from build123d import *

# Parameters (mm, degrees)
SKETCH1_W           = 190.5
SKETCH1_H           = 190.5
BOSS_EXTRUDE1_DEPTH = 9.525
SKETCH2_W           = 38.1
SKETCH2_H           = 9.525
CUT_EXTRUDE1_DEPTH  = 9.525
SKETCH3_W           = 38.1
SKETCH3_H           = 9.525
CUT_EXTRUDE2_DEPTH  = 9.525
SKETCH4_W           = 9.525
SKETCH4_H           = 28.575
CUT_EXTRUDE3_DEPTH  = 9.525
SKETCH5_W           = 9.525
SKETCH5_H           = 38.1
CUT_EXTRUDE4_DEPTH  = 9.525
SKETCH6_W           = 9.525
SKETCH6_H           = 28.575
CUT_EXTRUDE5_DEPTH  = 9.525
SKETCH7_W           = 38.1
SKETCH7_H           = 9.525
CUT_EXTRUDE6_DEPTH  = 9.525
SKETCH8_W           = 38.1
SKETCH8_H           = 9.525
CUT_EXTRUDE7_DEPTH  = 9.525
SKETCH9_W           = 9.525
SKETCH9_H           = 28.575
CUT_EXTRUDE8_DEPTH  = 38.1
SKETCH10_W          = 9.525
SKETCH10_H          = 38.1
CUT_EXTRUDE9_DEPTH  = 9.525
SKETCH11_W          = 9.525
SKETCH11_H          = 28.575
CUT_EXTRUDE10_DEPTH = 9.525
SKETCH12_W          = 25.4
SKETCH12_H          = 3.175
CUT_EXTRUDE11_DEPTH = 12.7
SKETCH15_W          = 6.35
SKETCH15_H          = 9.525
CUT_EXTRUDE14_DEPTH = 214.194785552
SKETCH19_W          = 6.35
SKETCH19_H          = 38.1
SKETCH19_H_2        = 9.525
CUT_EXTRUDE16_DEPTH = 214.194785552
SKETCH16_W          = 6.35
SKETCH16_H          = 38.1
SKETCH16_H_2        = 9.525
CUT_EXTRUDE15_DEPTH = 209.566482942


with BuildPart() as part:
    # Sketch1 → Boss-Extrude1 (new body)
    with BuildSketch(Plane(origin=(0, 0, 0), x_dir=(1, 0, 0), z_dir=(0, 1, 0))):
        with Locations((61.628840928, 48.799714441)):
            Rectangle(SKETCH1_W, SKETCH1_H)
    extrude(amount=BOSS_EXTRUDE1_DEPTH)

    # Sketch2 → Cut-Extrude1 (cut)
    with BuildSketch(Plane(origin=(0, 9.525, 0), x_dir=(1, 0, 0), z_dir=(0, 1, 0))):
        with Locations((99.728840928, -41.687785559)):
            Rectangle(SKETCH2_W, SKETCH2_H)
    extrude(amount=-CUT_EXTRUDE1_DEPTH, mode=Mode.SUBTRACT)

    # Sketch3 → Cut-Extrude2 (cut)
    with BuildSketch(Plane(origin=(0, 9.525, 0), x_dir=(1, 0, 0), z_dir=(0, 1, 0))):
        with Locations((23.528840928, -41.687785559)):
            Rectangle(SKETCH3_W, SKETCH3_H)
    extrude(amount=-CUT_EXTRUDE2_DEPTH, mode=Mode.SUBTRACT)

    # Sketch4 → Cut-Extrude3 (cut)
    with BuildSketch(Plane(origin=(0, 9.525, 0), x_dir=(1, 0, 0), z_dir=(0, 1, 0))):
        with Locations((152.116340928, -22.637785559)):
            Rectangle(SKETCH4_W, SKETCH4_H)
    extrude(amount=-CUT_EXTRUDE3_DEPTH, mode=Mode.SUBTRACT)

    # Sketch5 → Cut-Extrude4 (cut)
    with BuildSketch(Plane(origin=(0, 9.525, 0), x_dir=(1, 0, 0), z_dir=(0, 1, 0))):
        with Locations((152.116340928, 48.799714441)):
            Rectangle(SKETCH5_W, SKETCH5_H)
    extrude(amount=-CUT_EXTRUDE4_DEPTH, mode=Mode.SUBTRACT)

    # Sketch6 → Cut-Extrude5 (cut)
    with BuildSketch(Plane(origin=(0, 9.525, 0), x_dir=(1, 0, 0), z_dir=(0, 1, 0))):
        with Locations((152.116340928, 120.237214441)):
            Rectangle(SKETCH6_W, SKETCH6_H)
    extrude(amount=-CUT_EXTRUDE5_DEPTH, mode=Mode.SUBTRACT)

    # Sketch7 → Cut-Extrude6 (cut)
    with BuildSketch(Plane(origin=(0, 9.525, 0), x_dir=(1, 0, 0), z_dir=(0, 1, 0))):
        with Locations((99.728840928, 139.287214441)):
            Rectangle(SKETCH7_W, SKETCH7_H)
    extrude(amount=-CUT_EXTRUDE6_DEPTH, mode=Mode.SUBTRACT)

    # Sketch8 → Cut-Extrude7 (cut)
    with BuildSketch(Plane(origin=(0, 9.525, 0), x_dir=(1, 0, 0), z_dir=(0, 1, 0))):
        with Locations((23.528840928, 139.287214441)):
            Rectangle(SKETCH8_W, SKETCH8_H)
    extrude(amount=-CUT_EXTRUDE7_DEPTH, mode=Mode.SUBTRACT)

    # Sketch9 → Cut-Extrude8 (cut)
    with BuildSketch(Plane(origin=(0, 9.525, 0), x_dir=(1, 0, 0), z_dir=(0, 1, 0))):
        with Locations((-28.858659072, 120.237214441)):
            Rectangle(SKETCH9_W, SKETCH9_H)
    extrude(amount=-CUT_EXTRUDE8_DEPTH, mode=Mode.SUBTRACT)

    # Sketch10 → Cut-Extrude9 (cut)
    with BuildSketch(Plane(origin=(0, 9.525, 0), x_dir=(1, 0, 0), z_dir=(0, 1, 0))):
        with Locations((-28.858659072, 48.799714441)):
            Rectangle(SKETCH10_W, SKETCH10_H)
    extrude(amount=-CUT_EXTRUDE9_DEPTH, mode=Mode.SUBTRACT)

    # Sketch11 → Cut-Extrude10 (cut)
    with BuildSketch(Plane(origin=(0, 9.525, 0), x_dir=(1, 0, 0), z_dir=(0, 1, 0))):
        with Locations((-28.858659072, -22.637785559)):
            Rectangle(SKETCH11_W, SKETCH11_H)
    extrude(amount=-CUT_EXTRUDE10_DEPTH, mode=Mode.SUBTRACT)

    # Sketch12 → Cut-Extrude11 (cut)
    with BuildSketch(Plane(origin=(0, 9.525, 0), x_dir=(1, 0, 0), z_dir=(0, 1, 0))):
        with Locations((20.353840928, 101.187214441)):
            Rectangle(SKETCH12_W, SKETCH12_H)
        with Locations((102.903840928, 101.187214441)):
            Rectangle(SKETCH12_W, SKETCH12_H)
    extrude(amount=-CUT_EXTRUDE11_DEPTH, mode=Mode.SUBTRACT)

    # Sketch15 → Cut-Extrude14 (cut, through all)
    with BuildSketch(Plane(origin=(0, 9.525, 0), x_dir=(1, 0, 0), z_dir=(0, 1, 0))):
        with Locations((-30.446159072, 139.287214441)):
            Rectangle(SKETCH15_W, SKETCH15_H)
    extrude(amount=-CUT_EXTRUDE14_DEPTH, mode=Mode.SUBTRACT)

    # Sketch19 → Cut-Extrude16 (cut, through all)
    with BuildSketch(Plane(origin=(0, 9.525, 0), x_dir=(1, 0, 0), z_dir=(0, 1, 0))):
        with Locations((-30.446159072, 86.899714441)):
            Rectangle(SKETCH19_W, SKETCH19_H)
        with Locations((-30.446159072, 10.699714441)):
            Rectangle(SKETCH19_W, SKETCH19_H)
        with Locations((-30.446159072, -41.687785559)):
            Rectangle(SKETCH19_W, SKETCH19_H_2)
        with Locations((153.703840928, -41.687785559)):
            Rectangle(SKETCH19_W, SKETCH19_H_2)
        with Locations((153.703840928, 10.699714441)):
            Rectangle(SKETCH19_W, SKETCH19_H)
        with Locations((153.703840928, 86.899714441)):
            Rectangle(SKETCH19_W, SKETCH19_H)
        with Locations((153.703840928, 139.287214441)):
            Rectangle(SKETCH19_W, SKETCH19_H_2)
    extrude(amount=-CUT_EXTRUDE16_DEPTH, mode=Mode.SUBTRACT)

    # Sketch16 → Cut-Extrude15 (cut, through all)
    with BuildSketch(Plane(origin=(0, 9.525, 0), x_dir=(1, 0, 0), z_dir=(0, 1, 0))):
        with Locations((-30.446159072, 86.899714441)):
            Rectangle(SKETCH16_W, SKETCH16_H)
        with Locations((-30.446159072, 10.699714441)):
            Rectangle(SKETCH16_W, SKETCH16_H)
        with Locations((-30.446159072, -41.687785559)):
            Rectangle(SKETCH16_W, SKETCH16_H_2)
        with Locations((153.703840928, -41.687785559)):
            Rectangle(SKETCH16_W, SKETCH16_H_2)
        with Locations((153.703840928, 10.699714441)):
            Rectangle(SKETCH16_W, SKETCH16_H)
        with Locations((153.703840928, 86.899714441)):
            Rectangle(SKETCH16_W, SKETCH16_H)
        with Locations((153.703840928, 139.287214441)):
            Rectangle(SKETCH16_W, SKETCH16_H_2)
    extrude(amount=-CUT_EXTRUDE15_DEPTH, mode=Mode.SUBTRACT)


solid = part.part
Can you work these out from the model? Positions are in its coordinate system, mm. A direction names the side the tool comes from. Coordinates: 2 decimals unless noted, no trailing zeros. Write each loop counter-clockwise with the first axis right and the second up, starting at its lowest first coordinate (ties: lowest second). Pieces come first, ordered by that corner, then holes.
Q1. Imagine slicing it at C-C, the plane x = 86. List the corners of the cut face in (y, z) for me (3 decimals), plus the area to 3 significant figures.
Results found:
outline: (0, -134.525) - (9.525, -134.525) - (9.525, 36.925) - (0, 36.925) - close
area: 1,630 mm2
Q2. Please list where these lines run through material, in increasing order: L1, parallel to Z at x = 92, y = 6; L2, parallel to X at y = 8.5, z = 17; L3, parallel to Z at x = 84, y = 2.
Results found:
L1: z = -134.52 to -102.77, -99.6 to 36.93
L2: x = -24.1 to 147.35
L3: z = -134.52 to 36.93
Q3. Imagine slicing it at D-D, the plane z = -33. List the corners of the cut face in (x, y) for me (3 decimals).
Results found:
outline: (-24.096, 0) - (147.354, 0) - (147.354, 9.525) - (-24.096, 9.525) - close
Q4. If we mould it in two halves opening along X, with no side actions, what happens to faces 4 (the face through (134, 5, 46.45)), 5 (the face through (-24.096, 5, -49)), 6 (the face through (23, 5, 36.925))? For each: +X half, -X half, draft (parallel to the pull), parting line (faces both ways), or undercut.
Results found:
face 4: draft
face 5: -X half
face 6: undercut
Q5. Imagine slicing it at B-B, the plane y = 2. Count the separate pieces of the cut face and the enclosed holes in it, plus the area to 3 significant figures.
Results found:
separate pieces: 1
enclosed holes: 2
area: 31,700 mm2
Q6. For P1, Ø5, axis at y = 6, z = -39.5, coming from the +X side; P2, Ø3, axis at x = 107, y = 7.5, coming from the -Z side; P3, Ø3, axis at x = 107.5, y = 4, coming from the +Z side, each with a flat end and sliding along its axis, tell me the tip position at first contact or that it passes through.
Results found:
P1: stops at x = 147.35
P2: stops at z = -134.52
P3: stops at z = 36.93
Q7. Which directions (+Z, -Z, +X, -X, +Y, -Y) give clear straight access to the entire face, cutting with the end or side of a thin tool? Please do faces 1 (the face through (-24.096, 5, -120)), 2 (the face through (147.354, 5, -120)), 3 (the face through (99, 5, -134.525)).
Results found:
face 1: -X, +Y, -Y
face 2: +X, +Y, -Y
face 3: -Z, +Y, -Y
Q8. Imagine slicing it at A-A, the plane x = 16. List the corners of the cut face in (y, z) for me (3 decimals), plus the area to 3 significant figures.
Results found:
outline: (0, -134.525) - (9.525, -134.525) - (9.525, -102.775) - (0, -102.775) - close; (0, -99.6) - (9.525, -99.6) - (9.525, 36.925) - (0, 36.925) - close
area: 1,600 mm2
